Verification items for this drawing (mm, ordinates from the low corner). Round coordinates to 2 decimals unless told otherwise and drop trailing zeros. Loops run counter-clockwise (first coordinate to the right, second up) from the corner with the lowest first, then second, coordinate; pieces in that order, holes last. Notation, with made-up numbers: (39, -4) - (73, -4) arc R7 ccw to (73, 8) - close; hole circle Ø1 at (59.5, -21). An arc over 180 degrees is marked (long way). Put each result on its own line as item: value. Start each with the question number.
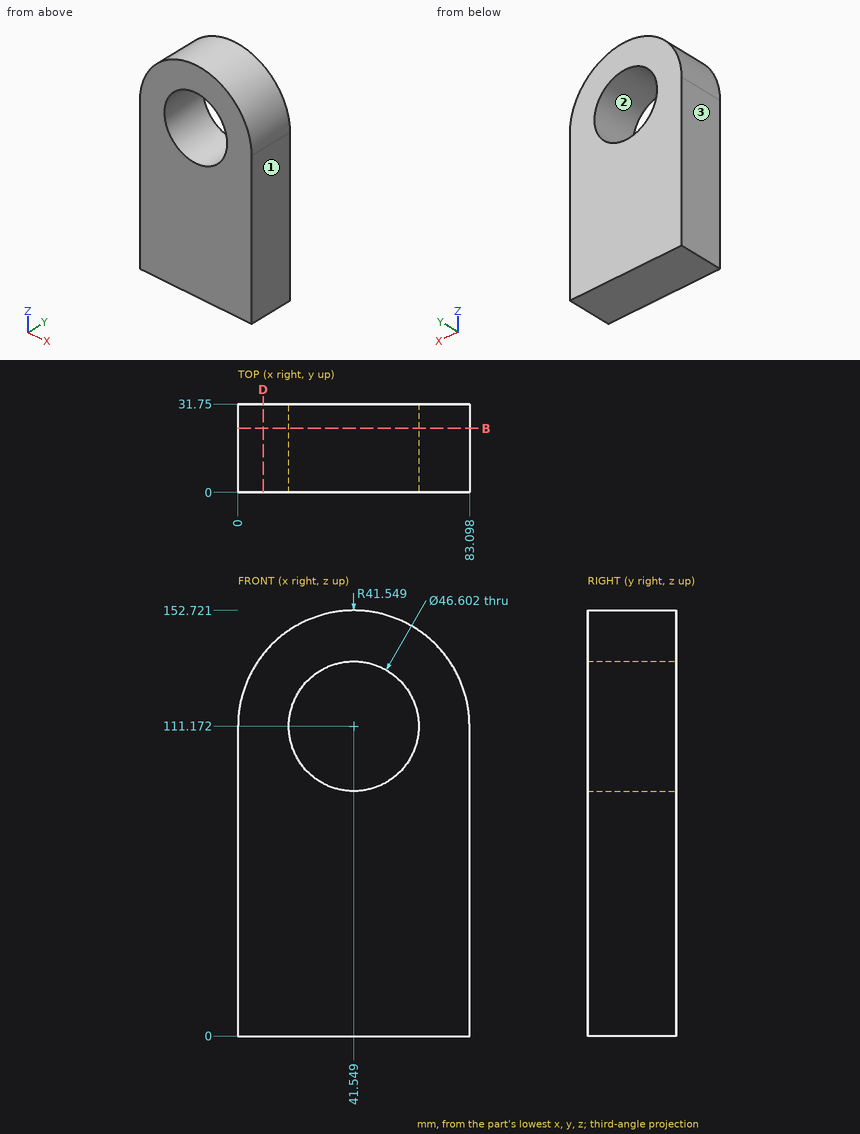
Q1. Cross-section at B-B on y = 23. Enter the section's corners in (x, z), and give its area (3 significant figures).
Q2. Material ranges on line 1 (Z direction, x = 60.5, y = 3.5) (1 decimal); line 2 (X direction, y = 29.5, z = 107.5); line 3 (Z direction, x = 26.5, y = 28.5), recorded low to high. Write a range as from..to.
Q3. Draft check along X on the marked faces 1, 2 and 3. Enter one of: +X half, -X half, draft (parallel to the pull), parting line (faces both ways), or undercut.
Q4. Cross-section at D-D on x = 9. Enter the section's corners in (y, z), and give its area (3 significant figures).
Q5. Depth check by flat-ended pin: pin 1 Ø1.5 at (x, y) = (54.5, 23.5) entering from +Z; pin 2 Ø10 at (x, y) = (56, 11) entering from +Z. Enter the tip coordinate at first touch or a pass-through.
Answer list:
1. outline: (0, 0) - (83.1, 0) - (83.1, 111.17) arc R41.55 ccw to (0, 111.17) - close; hole circle Ø46.6 at (41.55, 111.17)
1. area: 10,200 mm2
2. line 1: z = 0..97.6, 124.7..148.1
2. line 2: x = 0..18.54, 64.56..83.1
2. line 3: z = 0..93.38, 128.96..149.9
3. face 1: +X half
3. face 2: undercut
3. face 3: -X half
4. outline: (0, 0) - (31.75, 0) - (31.75, 137) - (0, 137) - close
4. area: 4,350 mm2
5. pin 1: stops at z = 150.89
5. pin 2: stops at z = 151.63
